Read the model definition and answer for the solid it produces. Units are mm, in the model's axes. A direction names the side the tool comes from. Give positions to 0.01 mm unless a question says otherwise; leave off trailing zeros. Loops run counter-clockwise (first coordinate to the right, second up) from the corner with the lowest first, then second, coordinate; pieces in that order, holes last. Notation, with made-up numbers: (-33, 52.5) -> (10, 52.5) arc R18 ccw to (10, 81.5) -> close; hole circle Ø2 at (51.5, -19.5). An arc over 180 degrees is marked (long way). Write each question's results on one line, items separated by ' | '. Start each with the question number.
Item 1: Section A-A on y = -133.35 is taken. Write down the section's boundary in (x, z), and give its area (3 significant figures).
Item 2: Determine the mould class of faces 1 (the cylindrical face through (-46.954, -136.998, -0.356)), 2 (the flat face through (-53.94, -161.09, 0.36)), 3 (the flat face through (-53, -101, -25.4)), 4 (the flat face through (29.3, 165.1, 9)) for opening direction Y: +Y half, -Y half, draft (parallel to the pull), parting line (faces both ways), or undercut.
Item 3: Section D-D on y = -16 is taken. Write down the section's boundary in (x, z), and give its area (3 significant figures).
Item 4: Each of these flat-tipped pins is pushed along its axis until it touches: P1, Ø2, axis at y = 23.5, z = -29, coming from the -X side; P2, Ø22, axis at x = -55.753, y = -133.35, coming from the -Z side; P3, Ø8, axis at y = 91, z = 13.5, coming from the +X side. Where does it stop, or does it pass through?
Item 5: Find the intervals of material crossed by line 1 (X direction, y = 22.5, z = 2); line 2 (X direction, y = -133, z = -6); line 3 (Z direction, x = 0, y = 92), in increasing order.
Item 6: Section C-C on x = -13.5 is taken. Write down the section's boundary in (y, z), and give its area (3 significant figures).
Item 7: Section B-B on z = -3 is taken. Write down the section's boundary in (x, y) (3 decimals).
Item 8: Which of the six approach directions +Z, -Z, +X, -X, +Y, -Y give full straight-line access (tool end or side, diameter ignored) to faces 5 (the flat face through (-53, -101, 25.4)), 6 (the cylindrical face through (42.687, 2.311, -5.605)), 7 (the cylindrical face through (-11.625, -2.311, 28.038))?
```python
from build123d import *

# Parameters (mm, degrees)
SKETCH1_R           = 43.053
SKETCH1_R_2         = 30.353
BOSS_EXTRUDE1_DEPTH = 165.1
SKETCH2_R           = 9.525
BOSS_EXTRUDE2_DEPTH = 25.4


with BuildPart() as part:
    # Sketch1 → Boss-Extrude1 (new, symmetric)
    with BuildSketch(Plane(origin=(0, 0, 0), x_dir=(1, 0, 0), z_dir=(0, 1, 0))):
        with Locations(Location((0, 0, 0), (0, 0, 270))):
            Circle(SKETCH1_R)
        with Locations(Location((0, 0, 0), (0, 0, 270))):
            Circle(SKETCH1_R_2, mode=Mode.SUBTRACT)
    extrude(amount=BOSS_EXTRUDE1_DEPTH, both=True)

    # Sketch2 → Boss-Extrude2 (add, symmetric)
    with BuildSketch(Plane.XY):
        with BuildLine():
            Line((-64.535931448, -157.183172579), (-43.053, -165.1))
            Line((-43.053, -165.1), (-30.353, -165.1))
            Line((-30.353, -165.1), (-30.353, 9.031002397))
            Line((-30.353, 9.031002397), (-79.586172579, -124.567068552))
            ThreePointArc((-79.586172579, -124.567068552), (-78.816068333, -143.992127562), (-64.535931448, -157.183172579))
        make_face()
        with Locations((-55.753, -133.35)):
            Circle(SKETCH2_R, mode=Mode.SUBTRACT)
    extrude(amount=BOSS_EXTRUDE2_DEPTH, both=True)


solid = part.part
```
Findings:
1) outline: (-81.15, -25.4) -> (-65.28, -25.4) -> (-65.28, 25.4) -> (-81.15, 25.4) -> close; (-46.23, -25.4) -> (-34.76, -25.4) arc R43.05 ccw (long way) to (-34.76, 25.4) -> (-46.23, 25.4) -> close; hole circle Ø60.71 at (0, 0) | area: 4,030 mm2
2) face 1: undercut | face 2: -Y half | face 3: draft | face 4: +Y half
3) outline: (-39.58, -25.4) -> (-34.76, -25.4) arc R43.05 ccw (long way) to (-34.76, 25.4) -> (-39.58, 25.4) -> (-39.58, 16.95) arc R43.05 ccw to (-39.58, -16.95) -> close; hole circle Ø60.71 at (0, 0) | area: 2,970 mm2
4) P1: x = -32.7 | P2: z = -25.4 | P3: x = 41.99
5) line 1: -43.01 to -30.29, 30.29 to 43.01 | line 2: -81.15 to -65.27, -46.23 to -29.75, 29.75 to 42.63 | line 3: -43.05 to -30.35, 30.35 to 43.05
6) outline: (-165.1, -40.88) -> (165.1, -40.88) -> (165.1, -27.19) -> (-165.1, -27.19) -> close; (-165.1, 27.19) -> (165.1, 27.19) -> (165.1, 40.88) -> (-165.1, 40.88) -> close | area: 9,040 mm2
7) outline: (-79.586, -124.567) arc R25.4 ccw to (-64.536, -157.183) -> (-43.053, -165.1) -> (-30.204, -165.1) -> (-30.204, 165.1) -> (-42.948, 165.1) -> (-42.948, -25.147) -> close; (30.204, -165.1) -> (42.948, -165.1) -> (42.948, 165.1) -> (30.204, 165.1) -> close; hole circle Ø19.05 at (-55.753, -133.35)
8) face 5: +Z, -X, +Y, -Y | face 6: +Y | face 7: +Y, -Y
